Geometry: final body of the model. Coordinates: model frame, mm. Face numbers are marked on the shaded views. A direction names the side the tool comes from. Round coordinates to 2 decimals unless told otherwise and drop trailing zeros. Loops run counter-clockwise (first coordinate to the right, second up) from the corner with the lowest first, then second, coordinate; pieces in that order, holes last. Notation, with made-up numbers: (76.25, 65.25) - (84.25, 65.25) arc R35 ccw to (84.25, 102.25) - close; hole circle Ø8 at (-16, 22.25). An arc over 180 degrees is marked (long way). Answer as a JSON object with one key per item and string values. Group by question number.
Item 1: Line query: line 1 (Y direction, x = 62.1, z = -6.25); line 2 (Y direction, x = 21.5, z = -3.5); line 3 (Y direction, x = 0, z = -4). Output: solid intervals per line, ascending.
Item 2: Section A-A (z = -0.5). Return the cut outline in (x, y), plus the area to 3 significant figures.
Item 3: Section B-B (x = 62.1). Return the cut outline in (y, z).
Item 4: Reachability of the marked faces 5, 6, 7, 8 and 9 from +Z, -Z, +X, -X, +Y, -Y: full face, straight path, thin tool, end or side. Return the list, or none.
Item 5: Section C-C (y = 0). Count the separate pieces of the cut face and the enclosed holes in it, plus the area to 3 significant figures.
Item 6: Draft query along Z for the marked faces 1, 2, 3 and 4. Return one class per face: released by +Z, released by -Z, zero draft, split by the parting line, or undercut.
Item 7: First-contact query: pin 1 (5 mm diameter, centred on x = 14.1, y = 5, fed in from +Z); pin 2 (6 mm diameter, centred on x = 107.5, y = 0.5, fed in from +Z); pin 3 (8 mm diameter, centred on y = -10.5, z = 7, fed in from +X). Flat tips, straight axial feed; report the tip coordinate or a pass-through.
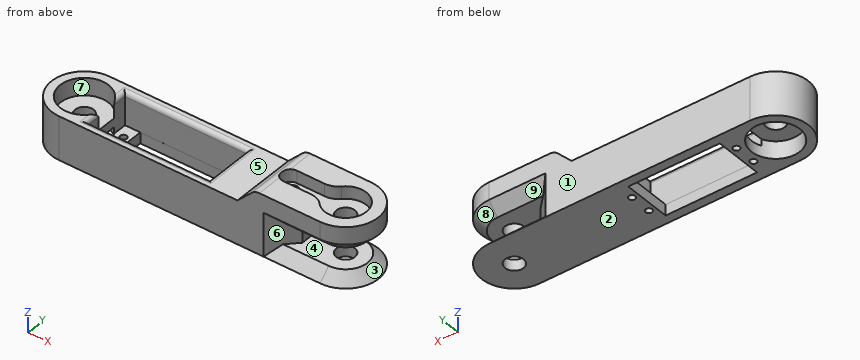
```python
from build123d import *

# Parameters (mm, degrees)
BOSS_EXTRUDE1_DEPTH = 10
SKETCH3_3_R         = 4.25
CUT_EXTRUDE5_DEPTH  = 12
SKETCH3_R           = 4.25
CUT_EXTRUDE6_DEPTH  = 138.295302177
SKETCH4_R           = 4.25
SKETCH4_W           = 42
SKETCH4_H           = 22
CUT_EXTRUDE8_DEPTH  = 138.295302177
SKETCH5_R           = 11.11
CUT_EXTRUDE10_DEPTH = 8
SKETCH7_W           = 56
SKETCH7_H           = 22.002715538
CUT_EXTRUDE12_DEPTH = 15
SKETCH8_R           = 1.5
CUT_EXTRUDE13_DEPTH = 14
SKETCH9_R           = 9.5
CUT_EXTRUDE14_DEPTH = 12
BOSS_EXTRUDE2_START = 8
SKETCH16_R          = 9.5
BOSS_EXTRUDE2_DEPTH = 8
CHAMFER1_SIZE       = 10
FILLET1_R           = 5
FILLET2_R           = 2
BOSS_EXTRUDE3_START = 14.3
SKETCH18_R          = 9.5
SKETCH18_R_2        = 4.25
BOSS_EXTRUDE3_DEPTH = 14.3
CUT_EXTRUDE15_DEPTH = 5.7
SKETCH19_R          = 2.155
CUT_EXTRUDE16_DEPTH = 6
CHAMFER2_SIZE       = 0.5
FILLET3_R           = 8
SKETCH20_W          = 31
SKETCH20_H          = 10
CUT_EXTRUDE17_DEPTH = 140.459671624
CHAMFER4_SIZE       = 5
CHAMFER5_SIZE       = 10


# Some blends are built 0.0001 mm under size
with BuildPart() as part:
    # Sketch1 → Boss-Extrude1 (new, symmetric)
    with BuildSketch(Plane.XY):
        with BuildLine():
            Line((120, 15), (0, 15))
            ThreePointArc((0, 15), (-15, 0), (0, -15))
            Line((0, -15), (120, -15))
            ThreePointArc((120, -15), (135, 0), (120, 15))
        make_face()
    extrude(amount=BOSS_EXTRUDE1_DEPTH, both=True)

    # Sketch3<3> → Cut-Extrude5 (cut)
    with BuildSketch(Plane.XY.offset(10)):
        with BuildLine():
            Line((120, 7.5), (118.514851485, 7.351485149))
            ThreePointArc((118.514851485, 7.351485149), (112.5, 0), (118.514851485, -7.351485149))
            Line((118.514851485, -7.351485149), (120, -7.5))
            ThreePointArc((120, -7.5), (125.303300859, -5.303300859), (127.5, 0))
            ThreePointArc((127.5, 0), (125.303300859, 5.303300859), (120, 7.5))
        make_face()
        with Locations((120, 0)):
            Circle(SKETCH3_3_R, mode=Mode.SUBTRACT)
    extrude(amount=-CUT_EXTRUDE5_DEPTH, mode=Mode.SUBTRACT)

    # Sketch3 → Cut-Extrude6 (cut, through all)
    with BuildSketch(Plane.XY.offset(10)):
        with Locations((120, 0)):
            Circle(SKETCH3_R)
    extrude(amount=-CUT_EXTRUDE6_DEPTH, mode=Mode.SUBTRACT)

    # Sketch4 → Cut-Extrude8 (cut, through all)
    with BuildSketch(Plane.XY.offset(10)):
        Circle(SKETCH4_R)
        with Locations((38.1, 0)):
            Rectangle(SKETCH4_W, SKETCH4_H)
    extrude(amount=-CUT_EXTRUDE8_DEPTH, mode=Mode.SUBTRACT)

    # Sketch5 → Cut-Extrude10 (cut)
    with BuildSketch(Plane(origin=(0, 0, -10), x_dir=(-1, 0, 0), z_dir=(0, 0, -1))):
        Circle(SKETCH5_R)
    cut_extrude10 = extrude(amount=-CUT_EXTRUDE10_DEPTH, mode=Mode.SUBTRACT)

    # Mirror2: Cut-Extrude10 across plane
    add(cut_extrude10.mirror(Plane.XY), mode=Mode.SUBTRACT)

    # Sketch7 → Cut-Extrude12 (cut)
    with BuildSketch(Plane.XY.offset(10)):
        with Locations((38.1, 0)):
            Rectangle(SKETCH7_W, SKETCH7_H)
    extrude(amount=-CUT_EXTRUDE12_DEPTH, mode=Mode.SUBTRACT)

    # Sketch8 → Cut-Extrude13 (cut)
    with BuildSketch(Plane.XY.offset(-5)):
        with Locations((14.1, 5)):
            Circle(SKETCH8_R)
        with Locations((14.1, -5)):
            Circle(SKETCH8_R)
        with Locations((62.1, -5)):
            Circle(SKETCH8_R)
        with Locations((62.1, 5)):
            Circle(SKETCH8_R)
    extrude(amount=-CUT_EXTRUDE13_DEPTH, mode=Mode.SUBTRACT)

    # Sketch9 → Cut-Extrude14 (cut)
    with BuildSketch(Plane.XY.offset(10)):
        with Locations((120, 0)):
            Circle(SKETCH9_R)
    extrude(amount=-CUT_EXTRUDE14_DEPTH, mode=Mode.SUBTRACT)

    # Sketch16 → Boss-Extrude2 (add)
    with BuildSketch(Plane.XY.offset(10).offset(BOSS_EXTRUDE2_START)):
        with BuildLine():
            ThreePointArc((120, -15), (135, 0), (120, 15))
            Line((120, 15), (80, 15))
            Line((80, 15), (80, -15))
            Line((80, -15), (120, -15))
        make_face()
        with Locations((120, 0)):
            Circle(SKETCH16_R, mode=Mode.SUBTRACT)
    extrude(amount=-BOSS_EXTRUDE2_DEPTH)

    # Chamfer1
    # the kernel refuses this chamfer: 10 mm, written as the material it takes off along each edge
    with BuildSketch(Plane(origin=(80, 40.71682988, 18), x_dir=(-0.027495876610586317, 0, -0.9996219169112968), z_dir=(0, -1, 0))) as chamfer1_piece_1_section:
        Polygon((CHAMFER1_SIZE * 0.999621916911, CHAMFER1_SIZE * 0.0274958766106), (-CHAMFER1_SIZE * 0.0274958766106, CHAMFER1_SIZE * 0.999621916911), (0, 0), align=None)
    chamfer1_piece_1 = extrude(amount=81.433659759, mode=Mode.PRIVATE)
    chamfer1_piece_1 = split(chamfer1_piece_1, bisect_by=Plane(origin=(83.457184123, 0, 10), z_dir=(0, 0, 1)), keep=Keep.TOP, mode=Mode.PRIVATE)
    add(chamfer1_piece_1, mode=Mode.SUBTRACT)

    # Fillet1
    fillet1_edges = [part.edges().sort_by_distance(p)[0] for p in [
        (90, 0, 18),
    ]]
    fillet(fillet1_edges, radius=FILLET1_R)

    # Fillet2
    fillet2_edges = [part.edges().sort_by_distance(p)[0] for p in [
        (10.1, -7.81487961, 10),
        (38.1, -11.001357769, 10),
        (66.1, 0, 10),
        (38.1, 11.001357769, 10),
        (10.1, 7.81487961, 10),
    ]]
    fillet(fillet2_edges, radius=FILLET2_R)

    # Sketch18 → Boss-Extrude3 (add)
    with BuildSketch(Plane.XY.offset(-2).offset(BOSS_EXTRUDE3_START)):
        with Locations((120, 0)):
            Circle(SKETCH18_R)
        with Locations((120, 0)):
            Circle(SKETCH18_R_2, mode=Mode.SUBTRACT)
    extrude(amount=-BOSS_EXTRUDE3_DEPTH)

    # Sketch17 → Cut-Extrude15 (cut)
    with BuildSketch(Plane.XY.offset(18)):
        with BuildLine():
            Line((113.07179677, -4), (94.5, -4))
            ThreePointArc((94.5, -4), (90.5, 0), (94.5, 4))
            Line((94.5, 4), (113.07179677, 4))
            ThreePointArc((113.07179677, 4), (128, 0), (113.07179677, -4))
        make_face()
    extrude(amount=-CUT_EXTRUDE15_DEPTH, mode=Mode.SUBTRACT)

    # Sketch19 → Cut-Extrude16 (cut)
    with BuildSketch(Plane.XY.offset(12.3)):
        with Locations((95.5, 0)):
            Circle(SKETCH19_R)
    extrude(amount=-CUT_EXTRUDE16_DEPTH, mode=Mode.SUBTRACT)

    # Chamfer2
    chamfer2_edges = [part.edges().sort_by_distance(p)[0] for p in [
        (93.345, 0, 12.3),
    ]]
    chamfer(chamfer2_edges, length=CHAMFER2_SIZE)

    # Fillet3
    fillet3_edges = [part.edges().sort_by_distance(p)[0] for p in [
        (111.38315603, 4, 15.15),
        (111.38315603, -4, 15.15),
    ]]
    fillet(fillet3_edges, radius=FILLET3_R)

    # Sketch20 → Cut-Extrude17 (cut, through all)
    with BuildSketch(Plane(origin=(0, 15, 0), x_dir=(1, 0, 0), z_dir=(0, 1, 0))):
        with Locations((119.5, 0)):
            Rectangle(SKETCH20_W, SKETCH20_H)
    extrude(amount=-CUT_EXTRUDE17_DEPTH, mode=Mode.SUBTRACT)

    # Chamfer4
    chamfer4_edges = [part.edges().sort_by_distance(p)[0] for p in [
        (112, 15, 5),
        (112, 15, -5),
        (135, 0, 5),
        (112, -15, 5),
        (135, 0, -5),
        (112, -15, -5),
    ]]
    chamfer(chamfer4_edges, length=CHAMFER4_SIZE - 0.0001)  # a hair under: the kernel refuses the full size

    # Chamfer5
    chamfer5_edges = [part.edges().sort_by_distance(p)[0] for p in [
        (104, 15, 0),
        (104, -15, 0),
    ]]
    chamfer(chamfer5_edges, length=CHAMFER5_SIZE)


solid = part.part
```
Values:
{
 "1": {"line 1": "y = -15 to -6.5, -3.5 to 3.5, 6.5 to 15", "line 2": "y = -15 to -11, 11 to 15", "line 3": "y = -15 to -11.11, 11.11 to 15"},
 "2": {"outline": "(0, -15) - (94, -15) - (104, -5) - (104, 5) - (94, 15) - (0, 15) arc R15 ccw to start; hole circle Ø8.5 at (0, 0); hole (10.1, -11) - (66.1, -11) - (66.1, 11) - (10.1, 11) - close", "area": "2,080 mm^2"},
 "3": {"outline": "(-15, -10) - (-6.5, -10) - (-6.5, -5) - (-11, -5) - (-11, 8) arc R2 ccw to (-13, 10) - (-15, 10) - close; (-3.5, -10) - (3.5, -10) - (3.5, -5) - (-3.5, -5) - close; (6.5, -10) - (15, -10) - (15, 10) - (13, 10) arc R2 ccw to (11, 8) - (11, -5) - (6.5, -5) - close"},
 "4": {"face 5": "+Z, -X, +Y, -Y", "face 6": "+X, -Y", "face 7": "+Z", "face 8": "+X", "face 9": "+X, +Y"},
 "5": {"separate pieces": "6", "enclosed holes": "0", "area": "1,270 mm^2"},
 "6": {"face 1": "zero draft", "face 2": "released by -Z", "face 3": "undercut", "face 4": "undercut"},
 "7": {"pin 1": "stops at z = -5", "pin 2": "stops at z = 12.3", "pin 3": "stops at x = 132.78"}
}
